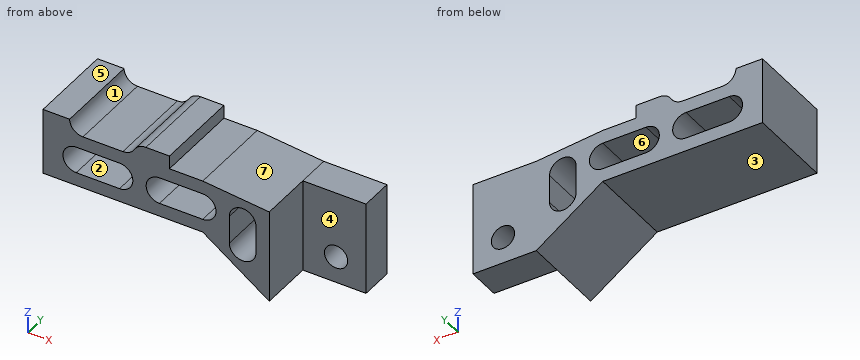
Autodesk Inventor part; units mm, degrees
ref_plane "YZ Plane" through (0, 0, 0) normal (1, 0, 0) x (0, 1, 0)
ref_plane "XZ Plane" through (0, 0, 0) normal (0, 1, 0) x (-1, 0, 0)
ref_plane "XY Plane" through (0, 0, 0) normal (0, 0, 1) x (1, 0, 0)
sketch "Sketch1" plane through (0, 0, 0) normal (0, 1, 0) x (-1, 0, 0)
  line L0 (15, 0) -> (15, 8)
  line L1 (15, 8) -> (20, 8)
  line L2 (20, 8) -> (20, 10)
  line L3 (20, 10) -> (25, 10)
  line L4 (25, 10) -> (25, 8)
  line L5 (25, 8) -> (35, 8)
  line L6 (35, 8) -> (35, 10)
  line L7 (35, 10) -> (39, 10)
  line L8 (39, 10) -> (39, 0)
  line L9 (39, 0) -> (15, 0)
  line L10 (15, 4) -> (39, 4)
  line L11 (39, 4) -> (34, 4)
  arc A0 (34, 2) -> (34, 6) centre (34, 4) ccw
  arc A1 (15, 6) -> (15, 2) centre (15, 4) ccw
  line L12 (34, 4) -> (15, 4)
  line L13 (24.5, 4) -> (27.5, 4)
  line L14 (24.5, 4) -> (21.5, 4)
  arc A2 (27.5, 6) -> (27.5, 2) centre (27.5, 4) ccw
  arc A3 (21.5, 2) -> (21.5, 6) centre (21.5, 4) ccw
  line L15 (15, 2) -> (21.5, 2)
  line L16 (27.5, 2) -> (34, 2)
  line L17 (15, 6) -> (21.5, 6)
  line L18 (27.5, 6) -> (34, 6)
  line L19 (5, 7) -> (15, 8)
  line L20 (5, 7) -> (-4.5, 7)
  line L21 (-4.5, 7) -> (-4.5, -3)
  line L22 (-4.5, -3) -> (0, -3)
  circle A4 centre (0, -3) radius 1.75
  line L23 (-4.5, -3) -> (-4.5, -7)
  line L24 (-4.5, -7) -> (5, -7)
  line L25 (5, -7) -> (5, 7)
  line L26 (5, -7) -> (15, 0)
  line L27 (5, 7) -> (9, 7)
  line L28 (9, 7) -> (9, 4)
  line L29 (9, -4.2) -> (9, -0.2)
  arc A5 (11, 4) -> (7, 4) centre (9, 4) ccw
  arc A6 (7, -0.2) -> (11, -0.2) centre (9, -0.2) ccw
  line L30 (7, 4) -> (7, -0.2)
  line L31 (11, -0.2) -> (11, 4)
  line L32 (9, 7) -> (9, 6)
  line L33 (9, -2.2) -> (9, -4.2)
  dimension "d6" = 8
  dimension "d7" = 5
  dimension "d8" = 2
  dimension "d9" = 5
  dimension "d10" = 2
  dimension "d11" = 10
  dimension "d12" = 2
  dimension "d13" = 4
  dimension "d15" = 5
  dimension "d16" = 4
  dimension "d17" = 4
  dimension "d18" = 3
  dimension "d19" = 3
  dimension "d20" = 4
  dimension "d21" = 4
  dimension "d36" = 10
  dimension "d37" = 4.5
  dimension "d38" = 3.5
  dimension "d39" = 4
  dimension "d40" = 4
  dimension "d41" = 3
  dimension "d42" = 4
  dimension "d43" = 4
  dimension "d44" = 4
extrude "Extrusion3" add sketch "Sketch1" against normal blind 8 contours L26 L29 A6 L31 A5 L28 L27 L19 L0 A1 | L0 L15 A3 L10 A2 L16 A0 L8 L9 | L26 L25 L27 L28 A5 L30 A6 L29 | L0 L1 L2 L3 L4 L5 L6 L7 L8 L10 A0 L18 A2 A3 L17
extrude "Extrusion4" add sketch "Sketch1" along normal blind 5 contours L26 L29 A6 L31 A5 L28 L27 L19 L0 A1 | L0 L15 A3 L10 A2 L16 A0 L8 L9 | L26 L25 L27 L28 A5 L30 A6 L29 | L0 L1 L2 L3 L4 L5 L6 L7 L8 L10 A0 L18 A2 A3 L17 | L24 L23 L21 L20 L25
fillet "Fillet2" radius 2 3 edges at (-25, -1.5, 8) (-25, -1.5, 10) (-35, -1.5, 8)
properties part number "servo_clip_header"
Geometry: final body of the model. Coordinates: model frame, mm. Face numbers are marked on the shaded views. A direction names the side the tool comes from. Round coordinates to 2 decimals unless told otherwise and drop trailing zeros. Order: outer loops, then holes, each group sorted by start corner. A loop starts at its lowest first (then second) coordinate and runs counter-clockwise, first axis right, second up. Notation, with made-up numbers: (-10, -27) - (49, -27) arc R20 ccw to (49, -19) - close; hole circle Ø11 at (33, -27). An arc over 180 degrees is marked (long way). Write item = value, one per line. Start each with the question number.
Q1. Pin query (flat end, axial travel): pin 1 (5 mm diameter, centred on x = -18, y = -2.5, fed in from -Z); pin 2 (1.5 mm diameter, centred on y = -2, z = 5.5, fed in from +X); pin 3 (1.5 mm diameter, centred on x = -1, y = 2, fed in from +Z). Return the tip coordinate at first contact, or that it passes through.
Q2. Access query for the marked faces 1, 2, 3 and 4. Directions: +Z, -Z, +X, -X, +Y, -Y. A direction counts if a zero-diameter tool reaches every point of the face in a straight line with its end or side. Return the directions, or none.
Q3. Cut plane C-C on x = -15.5. Return the cut outline in (y, z), and give its area (3 significant figures).
Q4. Pull-direction query (X, two-part tool) for the marked faces 5, 6 and 7; classes: +X half, -X half, draft (parallel to the pull), parting line (faces both ways), or undercut.
Q5. Ray query, line 1 (X direction, y = -4.5, z = 0.25); line 2 (Z direction, x = -29.5, y = -6.5); line 3 (Z direction, x = 0, y = 2). Return the intervals inside material, ascending. Write a range as from..to.
Q6. Cut plane D-D on z = 6.5. Return the cut outline in (x, y).
Q7. Cut plane B-B on z = -3. Return the cut outline in (x, y), and give its area (3 significant figures).
Q8. Cut plane A-A on x = 0. Return the cut outline in (y, z), and give its area (3 significant figures).
Outcome:
q1.pin_1 = 0
q1.pin_2 = -5
q1.pin_3 = 7
q2.face_1 = +Z, +Y, -Y
q2.face_2 = +Y, -Y
q2.face_3 = -Z, -X, +Y, -Y
q2.face_4 = +Z, -Z, +X, -Y
q3.outline = (-8, 0) - (5, 0) - (5, 2) - (-8, 2) - close; (-8, 6) - (5, 6) - (5, 8) - (-8, 8) - close
q3.area = 52.0 mm^2
q4.face_5 = draft
q4.face_6 = undercut
q4.face_7 = +X half
q5.line_1 = -39..-11, -7..-5
q5.line_2 = 0..2, 6..8
q5.line_3 = -7..-4.75, -1.25..7
q6.outline = (-39, -8) - (-5, -8) - (-5, 0) - (4.5, 0) - (4.5, 5) - (-39, 5) - close
q7.outline = (-10.71, -8) - (-5, -8) - (-5, 0) - (-1.75, 0) - (-1.75, 5) - (-10.71, 5) - close; (1.75, 0) - (4.5, 0) - (4.5, 5) - (1.75, 5) - close
q7.area = 104 mm^2
q8.outline = (0, -7) - (5, -7) - (5, -4.75) - (0, -4.75) - close; (0, -1.25) - (5, -1.25) - (5, 7) - (0, 7) - close
q8.area = 52.5 mm^2
